```python
from build123d import *

# Parameters (mm, degrees)
SKETCH1_W           = 150
SKETCH1_H           = 150
BOSS_EXTRUDE1_DEPTH = 19
SKETCH2_R           = 28
CUT_EXTRUDE1_DEPTH  = 3
SKETCH3_R           = 2.5
CUT_EXTRUDE2_DEPTH  = 5
CIRPATTERN1_COUNT   = 3
CIRPATTERN1_ANGLE   = 180


with BuildPart() as part:
    # Sketch1 → Boss-Extrude1 (new body)
    with BuildSketch(Plane(origin=(0, 0, 0), x_dir=(1, 0, 0), z_dir=(0, 1, 0))):
        with Locations((75, 75)):
            Rectangle(SKETCH1_W, SKETCH1_H)
    extrude(amount=BOSS_EXTRUDE1_DEPTH)

    # Sketch2 → Cut-Extrude1 (cut)
    with BuildSketch(Plane(origin=(0, 19, 0), x_dir=(1, 0, 0), z_dir=(0, 1, 0))):
        with Locations((75, 75)):
            Circle(SKETCH2_R)
    extrude(amount=-CUT_EXTRUDE1_DEPTH, mode=Mode.SUBTRACT)

    # Sketch3 → Cut-Extrude2 (cut)
    with BuildSketch(Plane(origin=(0, 19, 0), x_dir=(1, 0, 0), z_dir=(0, 1, 0))):
        with Locations((100, 5)):
            Circle(SKETCH3_R)
        with Locations((50, 5)):
            Circle(SKETCH3_R)
    cut_extrude2 = extrude(amount=-CUT_EXTRUDE2_DEPTH, mode=Mode.SUBTRACT)

    # CirPattern1: Cut-Extrude2 ×3 about axis
    cirpattern1_axis = Axis((75, 0, -75), (0, 1, 0))
    for i in range(1, CIRPATTERN1_COUNT):
        add(cut_extrude2.rotate(cirpattern1_axis, i * CIRPATTERN1_ANGLE / (CIRPATTERN1_COUNT - 1)), mode=Mode.SUBTRACT)


solid = part.part
```
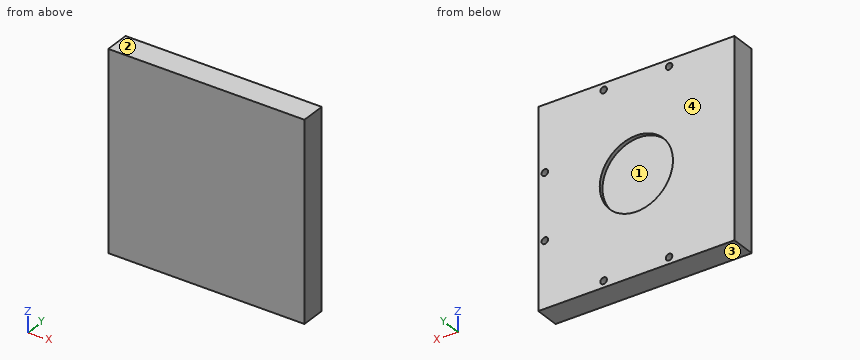
Could you check a few things on this model? Use its own coordinates, in mm. Face numbers are marked on the shaded views. Round coordinates to 2 decimals unless told otherwise and drop trailing zeros. Loops run counter-clockwise (first coordinate to the right, second up) from the corner with the lowest first, then second, coordinate; pieces in that order, holes last. Notation, with made-up numbers: M -31,3 L 21,3 A24 cw 21,29 Z; hole C 30.5,-9 d5. An arc over 180 degrees is marked long. Put each result on its own line as item: value.
Q1. Imagine slicing it at C-C (x = 70). Write out the boundary of the cut face in (y, z).
Check result:
outline: M 0,-150 L 19,-150 L 19,-102.55 L 16,-102.55 L 16,-47.45 L 19,-47.45 L 19,0 L 0,0 Z
Q2. I need wall thicknesses on probe 1 along Z at (x, y) = (145, 17.5); probe 2 along Z at (x, y) = (100, 15.9); probe 3 along Z at (x, y) = (50, 16.55). Which ranges of each line are inside material? Lowest first, please.
Check result:
probe 1: -150 to -102.5, -97.5 to -52.5, -47.5 to 0
probe 2: -150 to -147.5, -142.5 to -7.5, -2.5 to 0
probe 3: -150 to -147.5, -142.5 to -87.61, -62.39 to -7.5, -2.5 to 0
Q3. Imagine slicing it at A-A (x = 145). Write out the boundary of the cut face in (y, z), then the cut area to 3 significant figures.
Check result:
outline: M 0,-150 L 19,-150 L 19,-102.5 L 14,-102.5 L 14,-97.5 L 19,-97.5 L 19,-52.5 L 14,-52.5 L 14,-47.5 L 19,-47.5 L 19,0 L 0,0 Z
area: 2,800 mm2
Q4. Thinking about a two-plate mould opening in Z: for the marked faces 1, 2, 3 and 4, which applies, released by +Z, released by -Z, zero draft, split by the parting line, or undercut?
Check result:
face 1: undercut
face 2: released by +Z
face 3: released by -Z
face 4: zero draft
Q5. For pin 1 (1.5 mm diameter, centred on x = 51, z = -5, fed in from +Y); pin 2 (6 mm diameter, centred on x = 92, z = -90, fed in from +Y), each with a flat end and sliding along its axis, tell me the tip position at first contact or that it passes through.
Check result:
pin 1: y = 14
pin 2: y = 16
Q6. Imagine slicing it at B-B (z = -5). Write out the boundary of the cut face in (x, y), then the cut area to 3 significant figures.
Check result:
outline: M 0,0 L 150,0 L 150,19 L 102.5,19 L 102.5,14 L 97.5,14 L 97.5,19 L 52.5,19 L 52.5,14 L 47.5,14 L 47.5,19 L 0,19 Z
area: 2,800 mm2
Q7. Imagine slicing it at D-D (x = 100). Write out the boundary of the cut face in (y, z), then the cut area to 3 significant figures.
Check result:
outline: M 0,-150 L 19,-150 L 19,-147.5 L 14,-147.5 L 14,-142.5 L 19,-142.5 L 19,-87.61 L 16,-87.61 L 16,-62.39 L 19,-62.39 L 19,-7.5 L 14,-7.5 L 14,-2.5 L 19,-2.5 L 19,0 L 0,0 Z
area: 2,720 mm2
